Verification items for this drawing (mm, ordinates from the low corner). A direction names the side the tool comes from. Round coordinates to 2 decimals unless told otherwise and drop trailing zeros. Order: outer loops, then holes, each group sorted by start corner. A loop starts at its lowest first (then second) coordinate and runs counter-clockwise, first axis right, second up. Notation, with made-up numbers: (0, -19) -> (18, -19) arc R25 cw to (18, 1) -> close; hole circle Ø2 at (-0.5, 69). An arc over 180 degrees is marked (long way). Answer in a Markdown table with one row per item.
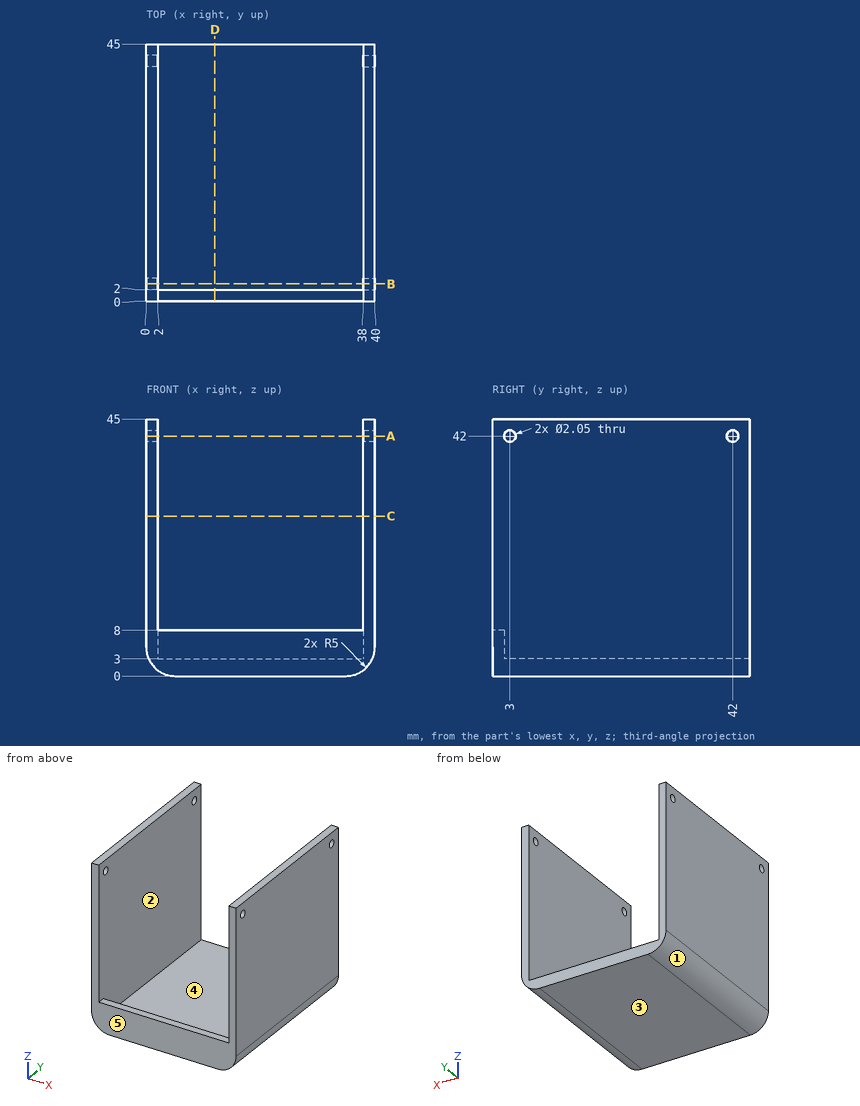
Item 1: Cross-section at A-A (z = 42). Record the boundary of the cut face in (x, y) (3 decimals).
Result sheet:
| item | result |
|---|---|
| outline | (0, 0) -> (2, 0) -> (2, 1.975) -> (0, 1.975) -> close; (0, 4.025) -> (2, 4.025) -> (2, 40.975) -> (0, 40.975) -> close; (0, 43.025) -> (2, 43.025) -> (2, 45) -> (0, 45) -> close; (38, 0) -> (40, 0) -> (40, 1.975) -> (38, 1.975) -> close; (38, 4.025) -> (40, 4.025) -> (40, 40.975) -> (38, 40.975) -> close; (38, 43.025) -> (40, 43.025) -> (40, 45) -> (38, 45) -> close |
Item 2: Cross-section at C-C (z = 28). Record the boundary of the cut face in (x, y), and give its area (3 significant figures).
Result sheet:
| item | result |
|---|---|
| outline | (0, 0) -> (2, 0) -> (2, 45) -> (0, 45) -> close; (38, 0) -> (40, 0) -> (40, 45) -> (38, 45) -> close |
| area | 180 mm^2 |
Item 3: Set-up check for the marked faces 4 and 5: record each of +Z, -Z, +X, -X, +Y, -Y from which the full face is reachable in a straight line by a thin tool's end or side.
Result sheet:
| item | result |
|---|---|
| face 4 | +Z, +Y |
| face 5 | +Z, -Z, +X, -X, -Y |
Item 4: Cross-section at D-D (x = 12). Record the boundary of the cut face in (y, z).
Result sheet:
| item | result |
|---|---|
| outline | (0, 0) -> (45, 0) -> (45, 3) -> (2, 3) -> (2, 8) -> (0, 8) -> close |
Item 5: Scan lines: line 1 (Y direction, x = 39, z = 42) (3 decimals); line 2 (X direction, y = 4, z = 6.5); line 3 (Z direction, x = 18.5, y = 23.5). Record each from-to range of solid material in increasing order. Write a range as [from, to].
Result sheet:
| item | result |
|---|---|
| line 1 | y = [0, 1.975], [4.025, 40.975], [43.025, 45] |
| line 2 | x = [0, 2], [38, 40] |
| line 3 | z = [0, 3] |
Item 6: Cross-section at B-B (y = 3). Record the boundary of the cut face in (x, z) (3 decimals).
Result sheet:
| item | result |
|---|---|
| outline | (0, 5) arc R5 ccw to (5, 0) -> (35, 0) arc R5 ccw to (40, 5) -> (40, 40.975) -> (38, 40.975) -> (38, 3) -> (2, 3) -> (2, 40.975) -> (0, 40.975) -> close; (0, 43.025) -> (2, 43.025) -> (2, 45) -> (0, 45) -> close; (38, 43.025) -> (40, 43.025) -> (40, 45) -> (38, 45) -> close |
Item 7: Mould release check, pull along X, two halves, no side actions. Record for the marked faces 1, 2 and 3: pulls with the +X half, pulls with the -X half, needs draft (parallel to the pull), parting line crosses it, or undercut.
Result sheet:
| item | result |
|---|---|
| face 1 | pulls with the -X half |
| face 2 | undercut |
| face 3 | needs draft |
Item 8: Depth check by flat-ended pin: P1, Ø6, axis at x = 19, y = 15.5, coming from the +Z side; P2, Ø1, axis at x = 24, y = 1, coming from the +Z side; P3, Ø2.5, axis at x = 21, z = 6, coming from the +Y side. Enter the tip coordinate at first touch or a pass-through.
Result sheet:
| item | result |
|---|---|
| P1 | stops at z = 3 |
| P2 | stops at z = 8 |
| P3 | stops at y = 2 |
